```python
from build123d import *

# Parameters (mm, degrees)
F1_DEPTH = 12.7


with BuildPart() as f1:
    # F0 (on Front) → F1 (new body)
    with BuildSketch(Plane.XZ):
        with BuildLine():
            Line((0, 25.4), (4.204138, 25.049655))
            ThreePointArc((4.204138, 25.049655), (2.109355, 25.312262), (0, 25.4))
        make_face()
        with BuildLine():
            Line((152.4, 12.7), (4.204138, 25.049655))
            Line((4.204138, 25.049655), (0, 25.4))
            ThreePointArc((0, 25.4), (-25.4, 0), (0, -25.4))
            Line((0, -25.4), (152.4, -12.7))
            ThreePointArc((152.4, -12.7), (165.1, 0), (152.4, 12.7))
        make_face()
        with BuildLine():
            ThreePointArc((0, 22.225), (1.845686, 22.148229), (3.678621, 21.918448))
            Line((3.678621, 21.918448), (152.4, 9.525))
            ThreePointArc((152.4, 9.525), (161.925, 0), (152.4, -9.525))
            Line((152.4, -9.525), (3.678621, -21.918448))
            ThreePointArc((3.678621, -21.918448), (1.845686, -22.148229), (0, -22.225))
            ThreePointArc((0, -22.225), (-22.225, 0), (0, 22.225))
        make_face(mode=Mode.SUBTRACT)
    extrude(amount=F1_DEPTH)


solid = f1.part
```
Design review of the part built by this model. Coordinates are the model's own, in mm. A direction names the side the tool comes from. Give positions to 0.01 mm unless a question says otherwise; leave off trailing zeros. Write each loop counter-clockwise with the first axis right and the second up, starting at its lowest first coordinate (ties: lowest second). Pieces come first, ordered by that corner, then holes. Notation, with made-up numbers: (-15, -34.75) -> (3, -34.75) arc R30 cw to (3, 0.25) -> close; hole circle Ø7 at (58.25, 43.5). An arc over 180 degrees is marked (long way). Answer in a Markdown table with one row per item.
(1) For faces 5 (the flat face through (79.34, -6.26, 18.79)), 6 (the cylindrical face through (161.923, -6.261, 0.209)), list the 3-axis set-ups (+Z, -Z, +X, -X, +Y, -Y) from which the entire face can be reached by the end or side of a thin tool; tool diameter is ignored.
Results:
| item | result |
|---|---|
| face 5 | +Z, +X, +Y, -Y |
| face 6 | +Y, -Y |
(2) Consider section B-B (y = -7). State the section outline as (x, z) points (3 decimals), then the cut area to 3 significant figures.
Results:
| item | result |
|---|---|
| outline | (0, -25.4) -> (152.4, -12.7) arc R12.7 ccw to (152.4, 12.7) -> (4.204, 25.05) arc R25.4 ccw to (0, 25.4) arc R25.4 ccw to start; hole (0, -22.225) arc R22.225 ccw to (3.679, -21.918) -> (152.4, -9.525) arc R9.525 ccw to (152.4, 9.525) -> (3.679, 21.918) arc R22.225 ccw to (0, 22.225) arc R22.225 ccw to start |
| area | 1,320 mm2 |
(3) Consider section A-A (z = 0). State the section outline as (x, y) points (3 decimals).
Results:
| item | result |
|---|---|
| outline | (-25.4, -12.7) -> (-22.225, -12.7) -> (-22.225, 0) -> (-25.4, 0) -> close; (161.925, -12.7) -> (165.1, -12.7) -> (165.1, 0) -> (161.925, 0) -> close |
(4) Mouldability with a two-part tool opening along X and no side actions: class faces 1 (the cylindrical face through (-22.22, -6.26, -0.49)), 2 (the cylindrical face through (-25.394, -6.261, 0.559)), 3 (the cylindrical face through (2.14, -6.26, 25.31)), 4 (the flat face through (77, -6.26, 15.81)) as +X half, -X half, draft (parallel to the pull), parting line (faces both ways), or undercut.
Results:
| item | result |
|---|---|
| face 1 | undercut |
| face 2 | -X half |
| face 3 | +X half |
| face 4 | undercut |
(5) To check wall thickness, follow probe 1 along Z at (x, y) = (55, -6.75); probe 2 along Z at (x, y) = (73, -5.5); probe 3 along X at (y, z) = (-2.25, 2.5). State the ranges of each line that lie inside material, in increasing order.
Results:
| item | result |
|---|---|
| probe 1 | -20.82 to -17.64, 17.64 to 20.82 |
| probe 2 | -19.32 to -16.14, 16.14 to 19.32 |
| probe 3 | -25.28 to -22.08, 161.59 to 164.85 |
(6) Clearance check with flat-ended pins moving along their axes: pin 1 (1 mm diameter, centred on y = -8, z = 1, fed in from +X); pin 2 (4 mm diameter, centred on y = -7, z = -6.5, fed in from -X); pin 3 (4 mm diameter, centred on y = -9, z = 16.5, fed in from -X). State where each tip first meets the part, or that it passes through.
Results:
| item | result |
|---|---|
| pin 1 | x = 165.09 |
| pin 2 | x = -25 |
| pin 3 | x = -20.85 |
(7) Consider section C-C (x = 65). State the section outline as (y, z) points, then the cut area to 3 significant figures.
Results:
| item | result |
|---|---|
| outline | (-12.7, -19.98) -> (0, -19.98) -> (0, -16.81) -> (-12.7, -16.81) -> close; (-12.7, 16.81) -> (0, 16.81) -> (0, 19.98) -> (-12.7, 19.98) -> close |
| area | 80.6 mm2 |
